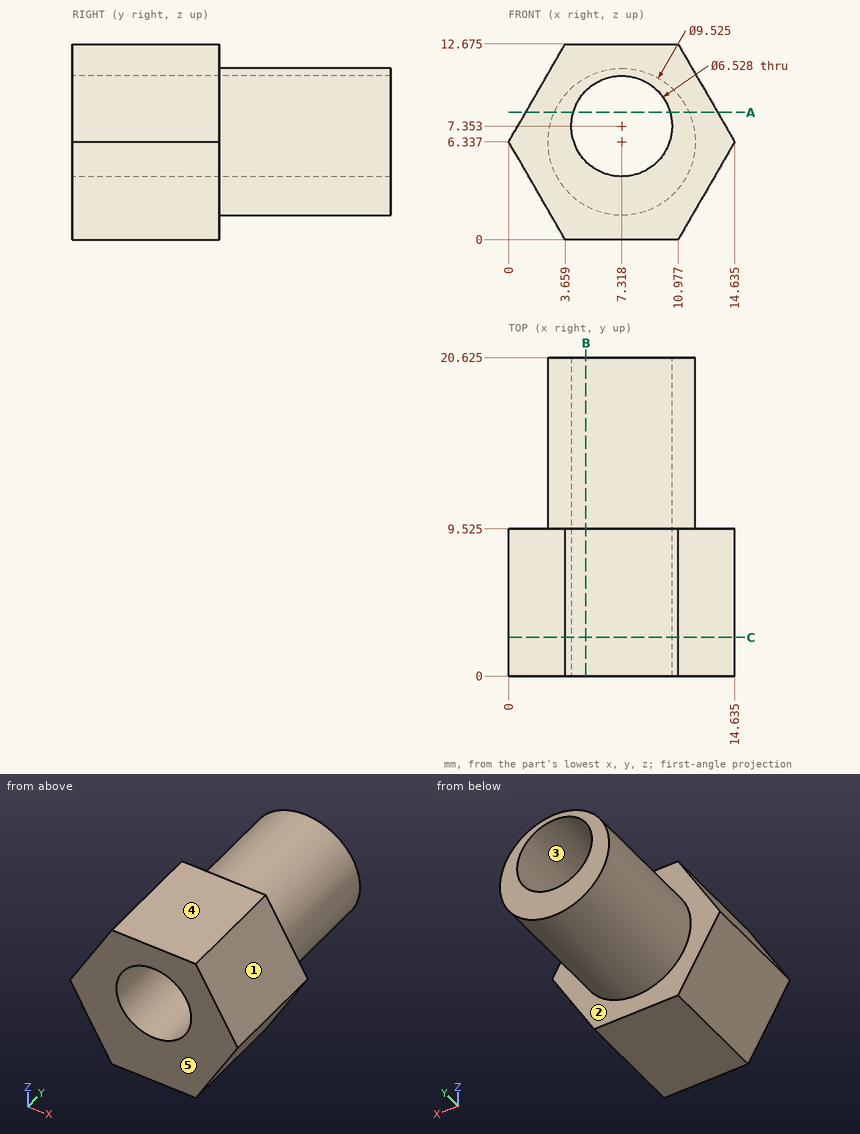
Can you work these out from the drawing? Everything is in mm from the part's minimum corner. A direction names the side the tool comes from. Coordinates: 2 decimals unless noted, no trailing zeros. Write each loop counter-clockwise with the first axis right and the second up, starting at its lowest first coordinate (ties: lowest second). Pieces come first, ordered by that corner, then holes. Notation, with made-up numbers: (67, 38) -> (96, 38) arc R15 cw to (96, 47) -> close; hole circle Ø5 at (-6, 29). An arc over 180 degrees is marked (long way). Write each question's results on one line, items separated by ' | '. Start each with the question number.
Item 1: On a 3-axis mill with a long thin cutter (end or side, diameter ignored), from which of +Z, -Z, +X, -X, +Y, -Y can I reach the whole of each face in a straight line? I mean the marked faces 1 and 2. Say none if no direction works.
Item 2: Thinking about a two-plate mould opening in Z: for the marked faces 3, 4 and 5, which applies, released by +Z, released by -Z, zero draft, split by the parting line, or undercut?
Item 3: If we section it at A-A, the plane z = 8.25: Write out the boundary of the cut face in (x, y) (1 decimal).
Item 4: Please list where these lines run through material, in increasing order: probe 1 along Y at (x, z) = (1.5, 5.75) (1 decimal); probe 2 along Z at (x, y) = (10.25, 13) (1 decimal); probe 3 along X at (y, z) = (16.25, 5) (1 decimal).
Item 5: If we section it at B-B, the plane x = 5: Write out the boundary of the cut face in (y, z) (1 decimal), and give its area (3 significant figures).
Item 6: If we section it at C-C, the plane y = 2.5: Write out the boundary of the cut face in (x, z) (1 decimal), and give its area (3 significant figures).
Item 7: I'm going to push flat-ended pins straight in: P1, Ø2, axis at y = 5, z = 9, coming from the +X side (1 decimal); P2, Ø3, axis at x = 11.5, y = 13, coming from the +Z side; P3, Ø4, axis at y = 2.5, z = 3.5, coming from the +X side. Where does each tip first touch, or does it pass through?
Answer block:
1) face 1: +Z, +X, +Y, -Y | face 2: +Y
2) face 3: undercut | face 4: released by +Z | face 5: zero draft
3) outline: (1.1, 0) -> (4.2, 0) -> (4.2, 20.6) -> (3, 20.6) -> (3, 9.5) -> (1.1, 9.5) -> close; (10.5, 0) -> (13.5, 0) -> (13.5, 9.5) -> (11.7, 9.5) -> (11.7, 20.6) -> (10.5, 20.6) -> close
4) probe 1: 0 to 9.5 | probe 2: 2.6 to 5.9, 8.8 to 10.1 | probe 3: 2.7 to 5.1, 9.6 to 11.9
5) outline: (0, 0) -> (9.5, 0) -> (9.5, 2.2) -> (20.6, 2.2) -> (20.6, 5.1) -> (0, 5.1) -> close; (0, 9.7) -> (20.6, 9.7) -> (20.6, 10.5) -> (9.5, 10.5) -> (9.5, 12.7) -> (0, 12.7) -> close | area: 118 mm²
6) outline: (0, 6.3) -> (3.7, 0) -> (11, 0) -> (14.6, 6.3) -> (11, 12.7) -> (3.7, 12.7) -> close; hole circle Ø6.5 at (7.3, 7.4) | area: 106 mm²
7) P1: x = 13.7 | P2: z = 10.27 | P3: x = 14.15
